Study the drawing (mm; zero at the part's minimum x, y, z) and answer. A direction names the side the tool comes from. Round coordinates to 2 decimals unless told otherwise and drop trailing zeros. Write each loop counter-clockwise with the first axis right and the second up, starting at its lowest first coordinate (ties: lowest second). Pieces come first, ordered by that corner, then holes. Notation, with made-up numbers: (-36, 54.25) - (-30, 54.25) arc R15 cw to (-30, 63.25) - close; hole circle Ø1 at (38.5, 66). An arc over 180 degrees is marked (long way). Use one line per item in the form item = value. Start each with the question number.
1) The part is cut by section B-B, the plane y = 10. Count the separate pieces of the cut face and the enclosed holes in it, plus the area to 3 significant figures.
2) The part is cut by section C-C, the plane z = 37.5. Give the vertices of the cut face in (x, y), plus the area to 3 significant figures.
3) Each of these flat-tipped pins is pushed along its axis until it touches: pin 1 (7.5 mm diameter, centred on x = 49, y = 6, fed in from +Z); pin 2 (10 mm diameter, centred on x = 40, z = 37, fed in from -Y); pin 3 (6 mm diameter, centred on y = 6, z = 23.5, fed in from +X); pin 4 (5 mm diameter, centred on y = 8.5, z = 45, fed in from -X). Where does it stop, or does it pass through?
4) For a pull along X with two mould halves and no side action, classify the marked faces 4, 5 and 6 as released by +X, released by -X, zero draft, split by the parting line, or undercut.
5) The part is cut by section A-A, the plane x = 7.5. Give the vertices of the cut face in (y, z), plus the area to 3 significant figures.
6) For the marked faces 1, 2 and 3, determine the directions among +Z, -Z, +X, -X, +Y, -Y from which every point of the face is accessible in a straight line to the end or side of a thin tool.
7) Consider line 1 along X through (y, z) = (10, 6); line 2 along Y through (x, z) = (7.5, 5.25); line 3 along X through (y, z) = (15.75, 31). Determine where each line is inside the solid, lowest interval first. Write a range as from..to.
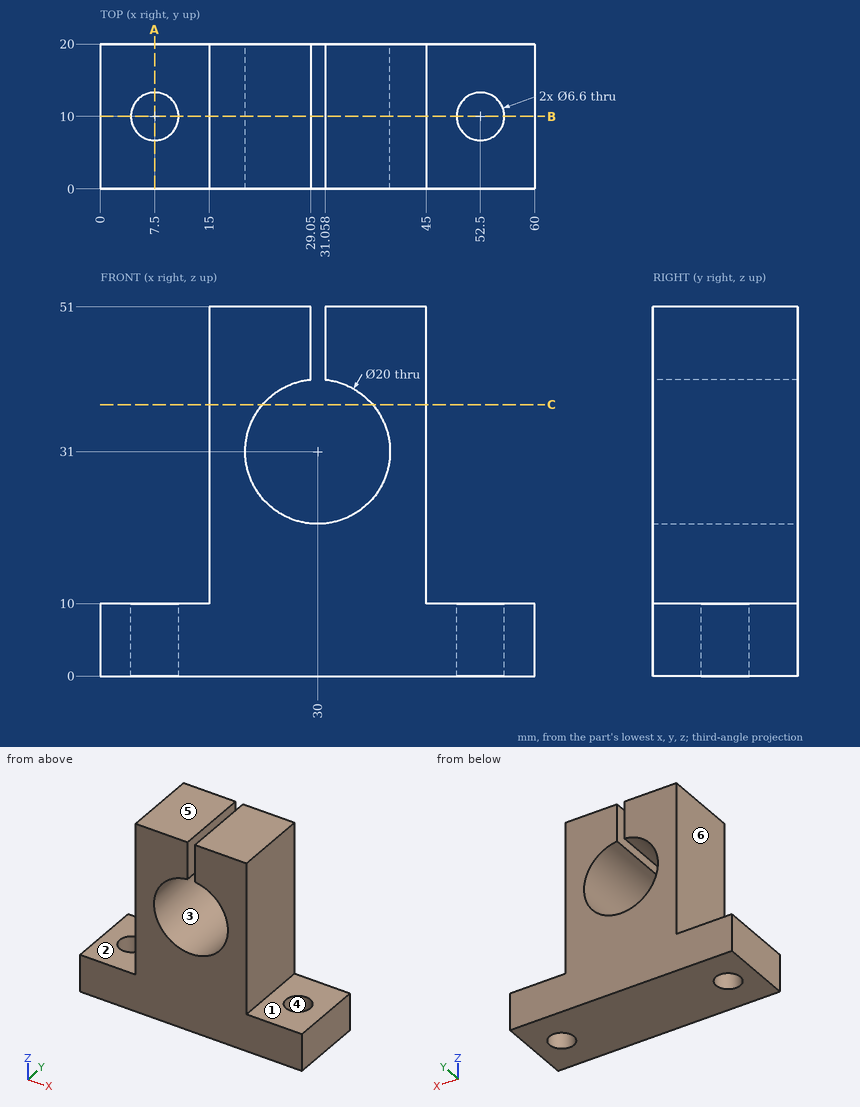
Geometry results:
q1.separate_pieces = 3
q1.enclosed_holes = 0
q1.area = 1,360 mm2
q2.outline = (15, 0) - (22.4, 0) - (22.4, 20) - (15, 20) - close; (37.6, 0) - (45, 0) - (45, 20) - (37.6, 20) - close
q2.area = 296 mm2
q3.pin_1 = 10
q3.pin_2 = 0
q3.pin_3 = 45
q3.pin_4 = 15
q4.face_4 = undercut
q4.face_5 = zero draft
q4.face_6 = released by -X
q5.outline = (0, 0) - (6.7, 0) - (6.7, 10) - (0, 10) - close; (13.3, 0) - (20, 0) - (20, 10) - (13.3, 10) - close
q5.area = 134 mm2
q6.face_1 = +Z, +X, +Y, -Y
q6.face_2 = +Z, -X, +Y, -Y
q6.face_3 = +Y, -Y
q7.line_1 = 0..4.2, 10.8..49.2, 55.8..60
q7.line_2 = 0..6.7, 13.3..20
q7.line_3 = 15..20, 40..45
